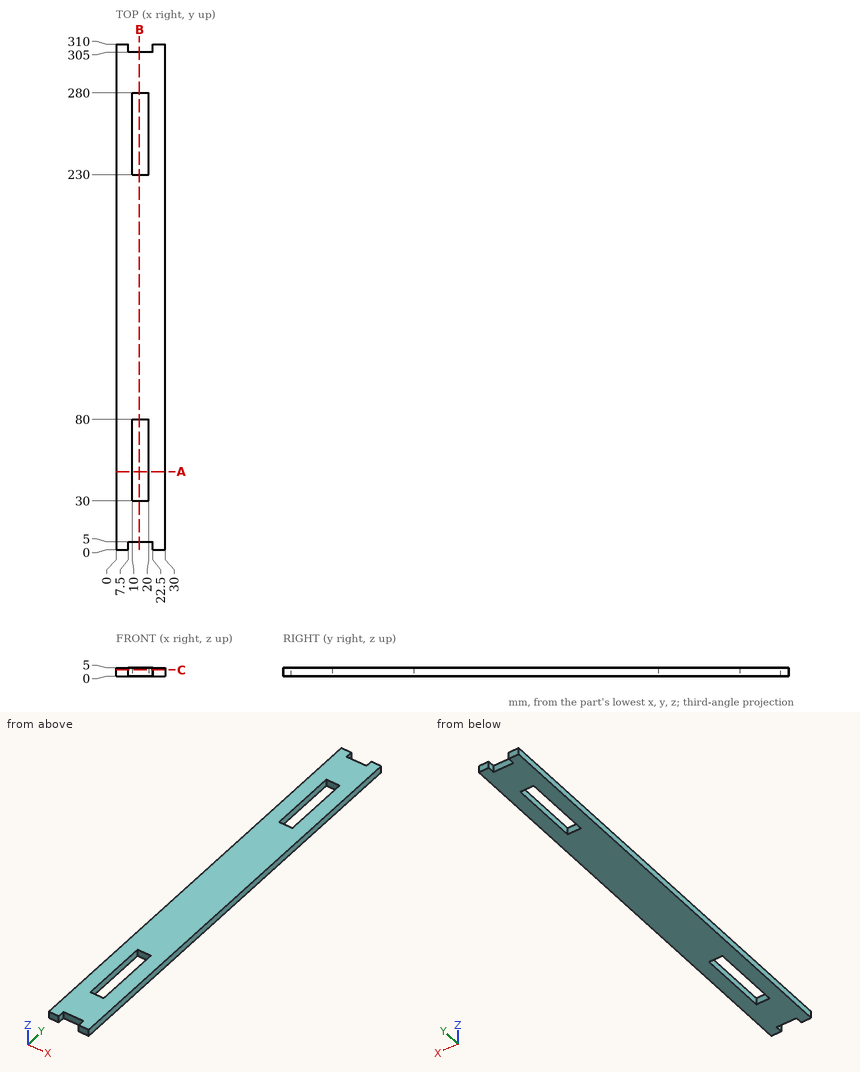
Answer from the drawing. Dimensions are ordinates in mm from the lowest x, y and z of the part. Give positions to 0.01 mm unless a question says otherwise; leave off trailing zeros. Write each loop counter-clockwise with the first axis right and the second up, starting at its lowest first coordinate (ties: lowest second). Pieces come first, ordered by that corner, then holes.
1) Find the intervals of material crossed by L1, parallel to Y at x = 19.75, z = 4; L2, parallel to X at y = 261.5, z = 3.35; L3, parallel to Y at x = 8.5, z = 4.1, in increasing order.
2) Given P1, Ø1.5, axis at x = 12, z = 2.5, coming from the -Y side; P2, Ø1.5, axis at x = 16, z = 3.5, coming from the +Y side, each flat-ended and moving along its own axis, determine where each tip first touches the part or whether it passes through.
3) Section B-B (x = 14.25) is taken. Write down the section's boundary in (y, z), and give its area (3 significant figures).
4) Section C-C (z = 3.7) is taken. Write down the section's boundary in (x, y), and give its area (3 significant figures).
5) Section A-A (y = 48) is taken. Write down the section's boundary in (x, z), and give its area (3 significant figures).
Response:
1. L1: y = 5 to 30, 80 to 230, 280 to 305
1. L2: x = 0 to 10, 20 to 30
1. L3: y = 5 to 305
2. P1: stops at y = 5
2. P2: stops at y = 305
3. outline: (5, 0) - (30, 0) - (30, 5) - (5, 5) - close; (80, 0) - (230, 0) - (230, 5) - (80, 5) - close; (280, 0) - (305, 0) - (305, 5) - (280, 5) - close
3. area: 1,000 mm2
4. outline: (0, 0) - (7.5, 0) - (7.5, 5) - (22.5, 5) - (22.5, 0) - (30, 0) - (30, 310) - (22.5, 310) - (22.5, 305) - (7.5, 305) - (7.5, 310) - (0, 310) - close; hole (10, 30) - (20, 30) - (20, 80) - (10, 80) - close; hole (10, 230) - (20, 230) - (20, 280) - (10, 280) - close
4. area: 8,150 mm2
5. outline: (0, 0) - (10, 0) - (10, 5) - (0, 5) - close; (20, 0) - (30, 0) - (30, 5) - (20, 5) - close
5. area: 100 mm2
